Read the model definition and answer for the solid it produces. Units are mm, in the model's axes. A direction names the side the tool comes from. Give positions to 0.01 mm unless a question says otherwise; leave off trailing zeros.
Item 1: Which of the six approach directions +Z, -Z, +X, -X, +Y, -Y give full straight-line access (tool end or side, diameter ignored) to faces 5 (the face through (-9, -28, -1)), 6 (the face through (-27.854, 0.676, -1.479)), 7 (the face through (-18, -0.1, 0.5)), 8 (the face through (9, 28, -1)), 9 (the face through (28, -8, 1))?
Item 2: A cutting plane is placed at A-A (y = -20). State how many separate pieces and enclosed holes the cut face has, plus the area to 3 significant figures.
Item 3: Find the intervals of material crossed by line 1 along Y through (x, z) = (0, -2.2); line 2 along Y through (x, z) = (30, -1.75); line 3 along X through (y, z) = (19.5, 0.85), in increasing order.
Item 4: Given pin 1 Ø1.5 at (x, z) = (6, -1.5) entering from +Y, flat-ended and moving along its own axis, determine where the tip first touches the part or whether it passes through.
Item 5: The mould has two halves that part along X. Classify faces 1 (the face through (39, 28, -1)), 2 (the face through (-1, 7, -3)), 3 (the face through (-0.33, 22.52, 0.49)), 4 (the face through (-28.962, -21.996, -1.479)): +X half, -X half, draft (parallel to the pull), parting line (faces both ways), or undercut.
Autodesk Fusion 360 part; units mm, degrees
sketch "Esquisse1" plane through (0, 0, 0) normal (0, 0, 1) x (1, 0, 0)
  line L0 (40, -10) -> (-40, -10)
  line L1 (-40, -10) -> (-40, 10)
  line L2 (-40, 10) -> (40, 10)
  line L3 (40, 10) -> (40, -10)
  line L4 (40, -10) -> (-40, 10) construction
  line L5 (-40, -10) -> (40, 10) construction
  line L6 (-40, -10) -> (-20, -10)
  line L7 (-20, -10) -> (-20, 25)
  line L8 (-25, 30) -> (-35, 30)
  line L9 (-40, 25) -> (-40, -10)
  line L10 (-40, 10) -> (-20, 10)
  line L11 (-20, 10) -> (-20, -25)
  line L12 (-25, -30) -> (-35, -30)
  line L13 (-40, -25) -> (-40, 10)
  line L14 (40, -10) -> (20, -10)
  line L15 (20, -10) -> (20, 25)
  line L16 (25, 30) -> (35, 30)
  line L17 (40, 25) -> (40, -10)
  line L18 (40, 10) -> (20, 10)
  line L19 (20, 10) -> (20, -25)
  line L20 (25, -30) -> (35, -30)
  line L21 (40, -25) -> (40, 10)
  circle A0 centre (-30, 20) radius 2.25
  circle A1 centre (30, 20) radius 2.25
  circle A2 centre (-30, -20) radius 2.25
  circle A3 centre (30, -20) radius 2.25
  circle A4 centre (0, 0) radius 5
  circle A5 centre (-20, 10) radius 5
  circle A6 centre (20, 10) radius 5
  circle A7 centre (-20, -10) radius 5
  circle A8 centre (20, -10) radius 5
  circle A9 centre (-30, 0) radius 2.25
  circle A10 centre (30, 0) radius 2.25
  circle A11 centre (-30, 10) radius 2.25
  circle A12 centre (30, 10) radius 2.25
  circle A13 centre (-30, -10) radius 2.25
  circle A14 centre (30, -10) radius 2.25
  arc A15 (-25, -30) -> (-20, -25) centre (-25, -25) ccw
  arc A16 (-40, -25) -> (-35, -30) centre (-35, -25) ccw
  arc A17 (-35, 30) -> (-40, 25) centre (-35, 25) ccw
  arc A18 (-20, 25) -> (-25, 30) centre (-25, 25) ccw
  arc A19 (25, 30) -> (20, 25) centre (25, 25) ccw
  arc A20 (40, 25) -> (35, 30) centre (35, 25) ccw
  arc A21 (35, -30) -> (40, -25) centre (35, -25) ccw
  circle A22 centre (0, 0) radius 15
  arc A23 (20, -25) -> (25, -30) centre (25, -25) ccw
  line L22 (5, 30) -> (-5, 30)
  line L23 (-10, 25) -> (-10, -25)
  line L24 (-5, -30) -> (5, -30)
  line L25 (10, -25) -> (10, 25)
  circle A24 centre (0, 25) radius 2.25
  circle A25 centre (0, -25) radius 2.25
  circle A26 centre (0, -15) radius 2.25
  circle A27 centre (0, 15) radius 2.25
  arc A28 (-5, 30) -> (-10, 25) centre (-5, 25) ccw
  arc A29 (10, 25) -> (5, 30) centre (5, 25) ccw
  arc A30 (-10, -25) -> (-5, -30) centre (-5, -25) ccw
  arc A31 (5, -30) -> (10, -25) centre (5, -25) ccw
  circle A32 centre (-15, 0) radius 2.25
  circle A33 centre (15, 0) radius 2.25
  point P0 (-40, 30)
  point P1 (-40, -30)
  point P2 (40, 30)
  point P3 (40, -30)
  point P4 (-10, 30)
  point P5 (-10, -30)
  point P6 (10, -30)
  dimension "d1" = 80
  dimension "d2" = 20
  dimension "d3" = 20
  dimension "d4" = 40
  dimension "d5" = 20
  dimension "d6" = 40
  dimension "d7" = 20
  dimension "d8" = 40
  dimension "d9" = 20
  dimension "d10" = 40
  dimension "d11" = 4.5
  dimension "d12" = 4.5
  dimension "d13" = 4.5
  dimension "d14" = 4.5
  dimension "d15" = 10
  dimension "d16" = 10
  dimension "d17" = 10
  dimension "d18" = 10
  dimension "d19" = 10
  dimension "d20" = 4.5
  dimension "d21" = 4.5
  dimension "d22" = 4.5
  dimension "d23" = 4.5
  dimension "d24" = 4.5
  dimension "d25" = 4.5
  dimension "d28" = 5
  dimension "d29" = 30
  dimension "d30" = 5
  dimension "d31" = 20
  dimension "d32" = 60
  dimension "d33" = 4.5
  dimension "d34" = 4.5
  dimension "d35" = 4.5
  dimension "d36" = 4.5
  dimension "d37" = 5
  dimension "d38" = 5
  dimension "d39" = 5
  dimension "d40" = 5
  dimension "d41" = 4.5
  dimension "d42" = 4.5
extrude "Extrusion1" add sketch "Esquisse1" against normal blind 3 contours L0 L14 L19 L20 L21 A8 A14 A21 A23 | L0 L2 L3 L14 L15 L17 L18 L19 L21 A6 A8 A12 A14 | L2 L15 L16 L17 L18 A6 A12 A19 A20 | L0 L14 L19 A8 | L0 L14 L15 L19 A8 | L0 L19 A8 | L0 L15 L19 A8 | L0 L2 L15 L19 A6 A8 A22 A33 | L2 L15 L18 L19 A6 | L2 L15 L18 A6 | L2 L15 L19 A6 | L2 L15 A6 | L0 A22 L25 | L0 L2 A22 L25 A33 | L0 A22 L23 L25 A26 | L0 L2 L23 L25 | A22 L23 L24 L25 A26 A30 A31 | L2 A22 L25 | L0 A22 L23 | L0 L2 A22 L23 A32 | L2 A22 L23 L25 A27 | A22 L22 L23 L25 A27 A28 A29 | L0 L2 L7 L11 A5 A7 A22 A32 | L2 A22 L23 | L0 L11 A7 | L0 L7 L11 A7 | L0 L6 L11 A7 | L0 L6 L7 L11 A7 | L0 L1 L2 L6 L7 L9 L10 L11 L13 A5 A7 A11 A13 | L0 L6 L11 L12 L13 A7 A13 A15 A16 | L2 L7 L11 A5 | L2 L7 A5 | L2 L7 L10 L11 A5 | L2 L7 L10 A5 | L2 L7 L8 L9 L10 A5 A11 A17 A18
sketch "Esquisse2" plane through (0, 0, 0) normal (0, 0, 1) x (1, 0, 0)
  circle A0 centre (30, 10) radius 2.25
  circle A1 centre (0, -15) radius 2.25
  circle A2 centre (-30, 20) radius 2.25
  circle A3 centre (30, 20) radius 2.25
  circle A4 centre (0, -25) radius 2.25
  circle A5 centre (0, 25) radius 2.25
  circle A6 centre (-30, 10) radius 2.25
  circle A7 centre (30, 0) radius 2.25
  circle A8 centre (-30, 0) radius 2.25
  circle A9 centre (0, 0) radius 5
  circle A10 centre (30, -20) radius 2.25
  circle A11 centre (-30, -20) radius 2.25
  circle A12 centre (-30, -10) radius 2.25
  circle A13 centre (0, 15) radius 2.25
  circle A14 centre (-15, 0) radius 2.25
  circle A15 centre (15, 0) radius 2.25
  circle A16 centre (30, -10) radius 2.25
  arc A17 (-11.1803, -10) -> (-10, -11.1803) centre (0, 0) ccw
  line L0 (-10, -11.1803) -> (-10, -25)
  arc A18 (-10, -25) -> (-5, -30) centre (-5, -25) ccw
  line L1 (-5, -30) -> (5, -30)
  arc A19 (5, -30) -> (10, -25) centre (5, -25) ccw
  line L2 (10, -25) -> (10, -11.1803)
  arc A20 (10, -11.1803) -> (11.1803, -10) centre (0, 0) ccw
  line L3 (11.1803, -10) -> (15, -10)
  arc A21 (15, -10) -> (20, -15) centre (20, -10) ccw
  line L4 (20, -15) -> (20, -25)
  arc A22 (20, -25) -> (25, -30) centre (25, -25) ccw
  line L5 (25, -30) -> (35, -30)
  arc A23 (35, -30) -> (40, -25) centre (35, -25) ccw
  line L6 (40, -25) -> (40, 25)
  arc A24 (40, 25) -> (35, 30) centre (35, 25) ccw
  line L7 (35, 30) -> (25, 30)
  arc A25 (25, 30) -> (20, 25) centre (25, 25) ccw
  line L8 (20, 25) -> (20, 15)
  arc A26 (20, 15) -> (15, 10) centre (20, 10) ccw
  line L9 (15, 10) -> (11.1803, 10)
  arc A27 (11.1803, 10) -> (10, 11.1803) centre (0, 0) ccw
  line L10 (10, 11.1803) -> (10, 25)
  arc A28 (10, 25) -> (5, 30) centre (5, 25) ccw
  line L11 (5, 30) -> (-5, 30)
  arc A29 (-5, 30) -> (-10, 25) centre (-5, 25) ccw
  line L12 (-10, 25) -> (-10, 11.1803)
  arc A30 (-10, 11.1803) -> (-11.1803, 10) centre (0, 0) ccw
  line L13 (-11.1803, 10) -> (-15, 10)
  arc A31 (-15, 10) -> (-20, 15) centre (-20, 10) ccw
  line L14 (-20, 15) -> (-20, 25)
  arc A32 (-20, 25) -> (-25, 30) centre (-25, 25) ccw
  line L15 (-25, 30) -> (-35, 30)
  arc A33 (-35, 30) -> (-40, 25) centre (-35, 25) ccw
  line L16 (-40, 25) -> (-40, -25)
  arc A34 (-40, -25) -> (-35, -30) centre (-35, -25) ccw
  line L17 (-35, -30) -> (-25, -30)
  arc A35 (-25, -30) -> (-20, -25) centre (-25, -25) ccw
  line L18 (-20, -25) -> (-20, -15)
  arc A36 (-20, -15) -> (-15, -10) centre (-20, -10) ccw
  line L19 (-15, -10) -> (-11.1803, -10)
  circle A37 centre (0, 25) radius 2.5
  circle A38 centre (0, 25) radius 3
  circle A39 centre (0, 15) radius 2.5
  circle A40 centre (-15, 0) radius 2.5
  circle A41 centre (-30, 10) radius 3
  circle A42 centre (-30, 20) radius 2.5
  circle A43 centre (-30, 0) radius 2.5
  circle A44 centre (-30, -10) radius 2.5
  circle A45 centre (-30, -20) radius 2.5
  circle A46 centre (0, -15) radius 2.5
  circle A47 centre (0, -25) radius 2.5
  circle A48 centre (15, 0) radius 2.5
  circle A49 centre (30, 10) radius 2.5
  circle A50 centre (30, 20) radius 2.5
  circle A51 centre (30, 0) radius 2.5
  circle A52 centre (30, -10) radius 2.5
  circle A53 centre (30, -20) radius 2.5
  circle A54 centre (0, 15) radius 3
  circle A55 centre (-15, 0) radius 3
  circle A56 centre (-30, 0) radius 3
  circle A57 centre (-30, 10) radius 2.5
  circle A58 centre (-30, 20) radius 3
  circle A59 centre (-30, -10) radius 3
  circle A60 centre (-30, -20) radius 3
  circle A61 centre (0, -15) radius 3
  circle A62 centre (0, -25) radius 3
  circle A63 centre (15, 0) radius 3
  circle A64 centre (30, 20) radius 3
  circle A65 centre (30, 10) radius 3
  circle A66 centre (30, 0) radius 3
  circle A67 centre (30, -10) radius 3
  circle A68 centre (30, -20) radius 3
  circle A69 centre (0, 0) radius 5.5
  circle A70 centre (0, 0) radius 6
  dimension "d43" = 5
  dimension "d44" = 6
  dimension "d45" = 5
  dimension "d46" = 5
  dimension "d47" = 6
  dimension "d48" = 5
  dimension "d49" = 5
  dimension "d50" = 5
  dimension "d51" = 5
  dimension "d52" = 5
  dimension "d53" = 5
  dimension "d54" = 5
  dimension "d55" = 5
  dimension "d56" = 5
  dimension "d57" = 5
  dimension "d58" = 5
  dimension "d59" = 5
  dimension "d60" = 6
  dimension "d61" = 6
  dimension "d62" = 6
  dimension "d63" = 5
  dimension "d64" = 6
  dimension "d65" = 6
  dimension "d66" = 6
  dimension "d67" = 6
  dimension "d68" = 6
  dimension "d69" = 6
  dimension "d70" = 6
  dimension "d71" = 6
  dimension "d72" = 6
  dimension "d73" = 6
  dimension "d74" = 6
  dimension "d75" = 11
  dimension "d76" = 12
extrude "Extrusion2" add sketch "Esquisse2" along normal blind 1 contours A38 | A41 | A54 | A55 | A56 | A58 | A59 | A60 | A61 | A62 | A63 | A64 | A65 | A66 | A67 | A68 | A70
Response values:
1. face 5: +Z, -Z, -Y
1. face 6: +Z, -Z
1. face 7: +Z
1. face 8: +Z, -Z, +Y
1. face 9: +Z, +X, -X, +Y, -Y
2. separate pieces: 5
2. enclosed holes: 0
2. area: 155 mm2
3. line 1: y = -30 to -27.25, -22.75 to -17.25, -12.75 to -5, 5 to 12.75, 17.25 to 22.75, 27.25 to 30
3. line 2: y = -30 to -22.25, -17.75 to -12.25, -7.75 to -2.25, 2.25 to 7.75, 12.25 to 17.75, 22.25 to 30
3. line 3: x = -32.96 to -32.45, -27.55 to -27.04, 27.04 to 27.55, 32.45 to 32.96
4. pin 1: stops at y = 29.99
5. face 1: +X half
5. face 2: draft
5. face 3: undercut
5. face 4: undercut
